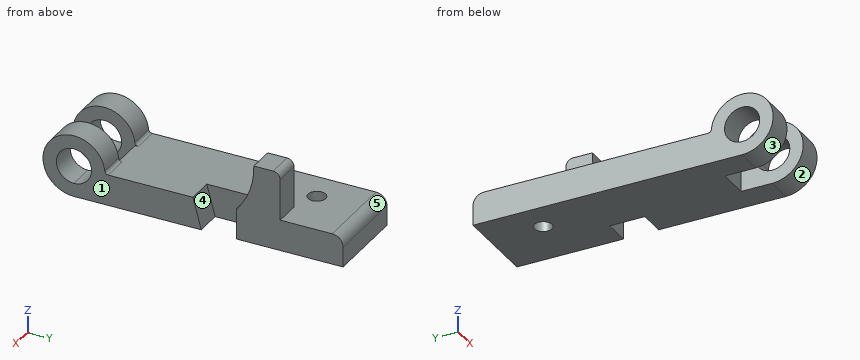
from build123d import *

# Parameters (mm, degrees)
F1_DEPTH  = 18.9992
F2_W      = 22.3266
F2_H      = 171.8564
F3_DEPTH  = 22.352
F5_R      = 12.7
F6_DEPTH  = 18.9992
F8_DEPTH  = 19.05
F10_DEPTH = 19.05
F11_R     = 6.35
F12_DEPTH = 22.353
F13_R     = 5.08
F14_R     = 7.874
F15_R     = 2.54


with BuildPart() as f1:
    # F0 (on Right) → F1 (new body)
    with BuildSketch(Plane.YZ):
        with BuildLine():
            ThreePointArc((22.352, 0), (-15.805251, 15.805251), (0, -22.352))
            Line((0, -22.352), (194.2084, -22.352))
            Line((194.2084, -22.352), (194.2084, 0))
            Line((194.2084, 0), (22.352, 0))
        make_face()
        with BuildLine():
            ThreePointArc((0, -12.7), (-8.980256, 8.980256), (12.7, 0))
            ThreePointArc((12.7, 0), (8.980256, -8.980256), (0, -12.7))
        make_face(mode=Mode.SUBTRACT)
    extrude(amount=-F1_DEPTH)

    # F2 (on Top) → F3 (join)
    with BuildSketch(Plane.XY):
        with Locations((-30.1625, 108.2802)):
            Rectangle(F2_W, F2_H)
    extrude(amount=-F3_DEPTH)

    # F5 (on offset) → F6 (join)
    with BuildSketch(Plane.YZ.offset(-41.3258)):
        with BuildLine():
            Line((194.2084, 0), (22.352, 0))
            ThreePointArc((22.352, 0), (-15.805251, 15.805251), (0, -22.352))
            Line((0, -22.352), (194.2084, -22.352))
            Line((194.2084, -22.352), (194.2084, 0))
        make_face()
        Circle(F5_R, mode=Mode.SUBTRACT)
    extrude(amount=-F6_DEPTH)

    # F7 (on Right) → F8 (cut)
    with BuildSketch(Plane.YZ):
        Polygon((117.2464, 0), (85.852, 0), (91.8464, -22.352), (117.2464, -22.352), align=None)
    extrude(amount=-F8_DEPTH, mode=Mode.SUBTRACT)

    # F9 (on Right) → F10 (join)
    with BuildSketch(Plane.YZ):
        with BuildLine():
            ThreePointArc((129.771803, 34.798), (126.921409, 16.24865), (117.530748, 0))
            Line((117.530748, 0), (148.821803, 0))
            Line((148.821803, 0), (148.821803, 34.798))
            Line((148.821803, 34.798), (129.771803, 34.798))
        make_face()
    extrude(amount=-F10_DEPTH)

    # F11 (on face) → F12 (cut, through all)
    with BuildSketch(Plane.XY):
        with Locations((-37.973, 155.3464)):
            Circle(F11_R)
    extrude(amount=-F12_DEPTH, mode=Mode.SUBTRACT)

    # F13
    f13_edges = [f1.edges().sort_by_distance(p)[0] for p in [
        (-9.525, 148.821803, 34.798),
    ]]
    fillet(f13_edges, radius=F13_R)

    # F14
    f14_edges = [f1.edges().sort_by_distance(p)[0] for p in [
        (-30.1625, 194.2084, 0),
    ]]
    fillet(f14_edges, radius=F14_R)

    # F15
    f15_edges = [f1.edges().sort_by_distance(p)[0] for p in [
        (-9.4996, 22.352, 0),
        (-50.8254, 22.352, 0),
    ]]
    fillet(f15_edges, radius=F15_R)


solid = f1.part
Read the model definition and answer for the solid it produces. Units are mm, in the model's axes. Face numbers are marked on the shaded views. A direction names the side the tool comes from. Coordinates: 2 decimals unless noted, no trailing zeros. Write each loop counter-clockwise with the first axis right and the second up, starting at its lowest first coordinate (ties: lowest second). Pieces come first, ordered by that corner, then holes. Notation, with made-up numbers: M 49.25,-20 L 108.25,-20 A13 ccw 108.25,-4 Z; hole C -9,-39 d9. An arc over 180 degrees is marked long. Use a Markdown table: item, result.
Q1. The part is cut by section C-C, the plane y = 10.5. Write down the section's boundary in (x, z) (3 decimals).
Answer block:
| item | result |
|---|---|
| outline | M -60.325,-22.352 L -41.326,-22.352 L -41.326,-7.144 L -60.325,-7.144 Z; M -60.325,7.144 L -41.326,7.144 L -41.326,19.732 L -60.325,19.732 Z; M -18.999,-22.352 L 0,-22.352 L 0,-7.144 L -18.999,-7.144 Z; M -18.999,7.144 L 0,7.144 L 0,19.732 L -18.999,19.732 Z |
Q2. Determine the mould class of the marked faces 1, 2 and 3 for opening direction Y: released by +Y, released by -Y, zero draft, split by the parting line, or undercut.
Answer block:
| item | result |
|---|---|
| face 1 | zero draft |
| face 2 | undercut |
| face 3 | split by the parting line |
Q3. The part is cut by section A-A, the plane x = -4. Write down the section's boundary in (y, z).
Answer block:
| item | result |
|---|---|
| outline | M 0,-22.35 L 91.85,-22.35 L 85.85,0 L 24.76,0 A2.54 cw 22.24,2.28 A22.35 ccw long Z; M 117.25,-22.35 L 194.21,-22.35 L 194.21,-7.87 A7.87 ccw 186.33,0 L 148.82,0 L 148.82,29.72 A5.08 ccw 143.74,34.8 L 129.77,34.8 A50.8 cw 117.53,0 L 117.25,0 Z; hole C 0,0 d25.4 |
Q4. Straight lines are drawn through the part: L1, parallel to Y at x = -8, z = -5; L2, parallel to Z at x = -54.5, y = 0; L3, parallel to Z at x = -31, y = 156. For each, find the intervals that lie inside material, in ascending order. Write a range as [from, to].
Answer block:
| item | result |
|---|---|
| L1 | y = [-21.79, -11.67], [11.67, 87.19], [117.25, 193.67] |
| L2 | z = [-22.35, -12.7], [12.7, 22.35] |
| L3 | z = [-22.35, 0] |
Q5. The part is cut by section D-D, the plane x = -51. Write down the section's boundary in (y, z).
Answer block:
| item | result |
|---|---|
| outline | M 0,-22.35 L 194.21,-22.35 L 194.21,-7.87 A7.87 ccw 186.33,0 L 24.76,0 A2.54 cw 22.24,2.28 A22.35 ccw long Z; hole C 0,0 d25.4 |
Q6. Each of these flat-tipped pins is pushed along its axis until it touches: pin 1 Ø23 at (y, z) = (0, 0) entering from -X; pin 2 Ø5 at (x, y) = (-21.5, 112) entering from +Z; pin 3 Ø6.5 at (y, z) = (101.5, -10.5) entering from +X; pin 4 Ø25 at (y, z) = (129, 20.5) entering from -X. Where does it stop, or does it pass through?
Answer block:
| item | result |
|---|---|
| pin 1 | passes through |
| pin 2 | stops at z = 0 |
| pin 3 | stops at x = -19.05 |
| pin 4 | stops at x = -19.05 |
Q7. Which of the six approach directions +Z, -Z, +X, -X, +Y, -Y give full straight-line access (tool end or side, diameter ignored) to the marked faces 4 and 5?
Answer block:
| item | result |
|---|---|
| face 4 | +Z, +X |
| face 5 | +Z, +X, -X, +Y |
Q8. The part is cut by section B-B, the plane z = 6. Write down the section's boundary in (x, y) (3 decimals), then the cut area to 3 significant figures.
Answer block:
| item | result |
|---|---|
| outline | M -60.325,-21.532 L -41.326,-21.532 L -41.326,-11.193 L -60.325,-11.193 Z; M -60.325,11.193 L -41.326,11.193 L -41.326,21.532 L -60.325,21.532 Z; M -19.05,121.964 L 0,121.964 L 0,148.822 L -19.05,148.822 Z; M -18.999,-21.532 L 0,-21.532 L 0,-11.193 L -18.999,-11.193 Z; M -18.999,11.193 L 0,11.193 L 0,21.532 L -18.999,21.532 Z |
| area | 1,300 mm2 |
